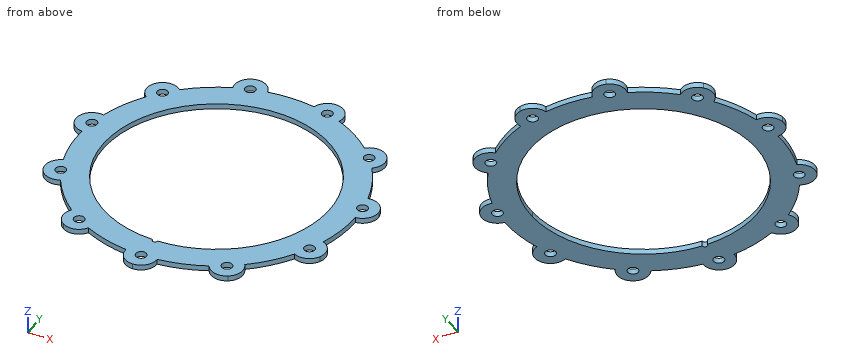
from build123d import *

# Parameters (mm, degrees)
SKETCH_1_R          = 42.7
SKETCH_1_R_2        = 2
EXTRUDE_1_DEPTH     = 2
SKETCH_2_R          = 1
CUT_EXTRUDE_1_DEPTH = 2


with BuildPart() as part:
    # 草图1 → 凸台-拉伸1 (new body)
    with BuildSketch(Plane.XY):
        with BuildLine():
            ThreePointArc((-70.701698086, -22.554916187), (-69.461279061, -27.140293833), (-65.275895868, -29.386823389))
            ThreePointArc((-65.275895868, -29.386823389), (-64.762769434, -38.351863236), (-62.729367044, -47.098320399))
            ThreePointArc((-62.729367044, -47.098320399), (-66.112292293, -50.433008431), (-66.010615464, -55.182112487))
            ThreePointArc((-66.010615464, -55.182112487), (-62.488066258, -58.368956475), (-57.752532286, -57.99606841))
            ThreePointArc((-57.752532286, -57.99606841), (-52.473996389, -65.260522759), (-46.034697694, -71.519170416))
            ThreePointArc((-46.034697694, -71.519170416), (-47.077727048, -76.153435976), (-44.424631557, -80.093665897))
            ThreePointArc((-44.424631557, -80.093665897), (-39.738336654, -80.870175779), (-35.956150478, -77.996259418))
            ThreePointArc((-35.956150478, -77.996259418), (-27.58810297, -81.253715341), (-18.787339807, -83.037477084))
            ThreePointArc((-18.787339807, -83.037477084), (-17.159318816, -87.4999736), (-12.797143736, -89.380334226))
            ThreePointArc((-12.797143736, -89.380334226), (-8.434968656, -87.4999736), (-6.806947664, -83.037477084))
            ThreePointArc((-6.806947664, -83.037477084), (1.993815499, -81.253715341), (10.361863007, -77.996259418))
            ThreePointArc((10.361863007, -77.996259418), (14.144049183, -80.870175779), (18.830344086, -80.093665897))
            ThreePointArc((18.830344086, -80.093665897), (21.483439576, -76.153435976), (20.440410223, -71.519170416))
            ThreePointArc((20.440410223, -71.519170416), (26.879708918, -65.260522759), (32.158244814, -57.99606841))
            ThreePointArc((32.158244814, -57.99606841), (36.893778787, -58.368956475), (40.416327993, -55.182112487))
            ThreePointArc((40.416327993, -55.182112487), (40.518004822, -50.433008431), (37.135079573, -47.098320399))
            ThreePointArc((37.135079573, -47.098320399), (39.168481963, -38.351863236), (39.681608397, -29.386823389))
            ThreePointArc((39.681608397, -29.386823389), (43.866991589, -27.140293833), (45.107410614, -22.554916187))
            ThreePointArc((45.107410614, -22.554916187), (42.625387107, -18.504744978), (37.976620826, -17.528374363))
            ThreePointArc((37.976620826, -17.528374363), (34.958536021, -9.071046044), (30.543338974, -1.251757506))
            ThreePointArc((30.543338974, -1.251757506), (32.849741796, 2.90093241), (31.414206364, 7.429018709))
            ThreePointArc((31.414206364, 7.429018709), (27.136507447, 9.49435633), (22.697850582, 7.802418757))
            ThreePointArc((22.697850582, 7.802418757), (15.586499181, 13.285476247), (7.644772521, 17.476444614))
            ThreePointArc((7.644772521, 17.476444614), (7.339928372, 22.216845183), (3.68421084, 25.25000473))
            ThreePointArc((3.68421084, 25.25000473), (-1.031024306, 24.67477866), (-3.850329562, 20.851711124))
            ThreePointArc((-3.850329562, 20.851711124), (-12.797143736, 21.619665774), (-21.743957909, 20.851711124))
            ThreePointArc((-21.743957909, 20.851711124), (-24.563263165, 24.67477866), (-29.278498311, 25.25000473))
            ThreePointArc((-29.278498311, 25.25000473), (-32.934215843, 22.216845183), (-33.239059992, 17.476444613))
            ThreePointArc((-33.239059992, 17.476444613), (-41.180786652, 13.285476247), (-48.292138053, 7.802418757))
            ThreePointArc((-48.292138053, 7.802418757), (-52.730794918, 9.49435633), (-57.008493835, 7.429018709))
            ThreePointArc((-57.008493835, 7.429018709), (-58.444029267, 2.90093241), (-56.137626446, -1.251757506))
            ThreePointArc((-56.137626446, -1.251757506), (-60.552823492, -9.071046044), (-63.570908298, -17.528374363))
            ThreePointArc((-63.570908298, -17.528374363), (-68.219674578, -18.504744978), (-70.701698086, -22.554916187))
        make_face()
        with Locations((-12.797143736, -30.880334226)):
            Circle(SKETCH_1_R, mode=Mode.SUBTRACT)
        with Locations((-64.762769434, -23.408805217)):
            Circle(SKETCH_1_R_2, mode=Mode.SUBTRACT)
        with Locations((-52.473996389, 3.499854306)):
            Circle(SKETCH_1_R_2, mode=Mode.SUBTRACT)
        with Locations((-27.58810297, 19.493046888)):
            Circle(SKETCH_1_R_2, mode=Mode.SUBTRACT)
        with Locations((1.993815499, 19.493046888)):
            Circle(SKETCH_1_R_2, mode=Mode.SUBTRACT)
        with Locations((26.879708918, 3.499854306)):
            Circle(SKETCH_1_R_2, mode=Mode.SUBTRACT)
        with Locations((39.168481963, -23.408805217)):
            Circle(SKETCH_1_R_2, mode=Mode.SUBTRACT)
        with Locations((34.958536021, -52.689622409)):
            Circle(SKETCH_1_R_2, mode=Mode.SUBTRACT)
        with Locations((15.586499181, -75.0461447)):
            Circle(SKETCH_1_R_2, mode=Mode.SUBTRACT)
        with Locations((-12.797143736, -83.380334226)):
            Circle(SKETCH_1_R_2, mode=Mode.SUBTRACT)
        with Locations((-41.180786652, -75.0461447)):
            Circle(SKETCH_1_R_2, mode=Mode.SUBTRACT)
        with Locations((-60.552823492, -52.689622409)):
            Circle(SKETCH_1_R_2, mode=Mode.SUBTRACT)
    extrude(amount=EXTRUDE_1_DEPTH)

    # 草图2 → 切除-拉伸1 (cut)
    with BuildSketch(Plane.XY.offset(2)):
        with Locations((-12.797143736, -73.580334226)):
            Circle(SKETCH_2_R)
    extrude(amount=-CUT_EXTRUDE_1_DEPTH, mode=Mode.SUBTRACT)


solid = part.part
The model under review builds one solid part; all positions refer to its coordinate system, in mm. Round coordinates to 2 decimals unless told otherwise and drop trailing zeros. Order: outer loops, then holes, each group sorted by start corner. A loop starts at its lowest first (then second) coordinate and runs counter-clockwise, first axis right, second up. Notation, with made-up numbers: (52, -10) -> (105, -10) arc R23 ccw to (105, 21) -> close; hole circle Ø11 at (13.5, 81.5). An arc over 180 degrees is marked (long way). Write item = value, one per line. Start each with the question number.
Item 1: Consider section A-A on x = 6. Write out the cut boundary in (y, z).
Item 2: Clearance check with flat-ended pins moving along their axes: pin 1 Ø2.5 at (x, y) = (-64.76, -23.41) entering from +Z; pin 2 Ø1 at (x, z) = (5.5, 0) entering from +Y; pin 3 Ø1 at (x, z) = (-36, 0.5) entering from +Y. State where each tip first meets the part, or that it passes through.
Item 3: Consider section C-C on z = 1. Count the separate pieces of the cut face and the enclosed holes in it, plus the area to 3 significant figures.
Item 4: For line 1 along X through (y, z) = (-25, 1.45); line 2 along X through (y, z) = (-78.5, 1.2); line 3 along Y through (x, z) = (-43, 1.4), list the stretches that pass through material, from the lowest coordinate up.
Item 5: Consider section B-B on y = -66. Write out the cut boundary in (x, z).
Conclusion:
q1.outline = (-79.9, 0) -> (-69.22, 0) -> (-69.22, 2) -> (-79.9, 2) -> close; (7.46, 0) -> (23.96, 0) -> (23.96, 2) -> (7.46, 2) -> close
q2.pin_1 = through
q2.pin_2 = 24.69
q2.pin_3 = 16.46
q3.separate_pieces = 1
q3.enclosed_holes = 12
q3.area = 3,430 mm2
q4.line_1 = -70.55 to -65.97, -63.55 to -55.09, 29.5 to 37.96, 40.38 to 44.95
q4.line_2 = -46.09 to -36.27, -34.9 to 9.31, 10.68 to 20.49
q4.line_3 = -80.76 to -75.88, -74.22 to -61.06, -0.7 to 12.06
q5.outline = (-51.82, 0) -> (-37.08, 0) -> (-37.08, 2) -> (-51.82, 2) -> close; (11.49, 0) -> (26.23, 0) -> (26.23, 2) -> (11.49, 2) -> close
